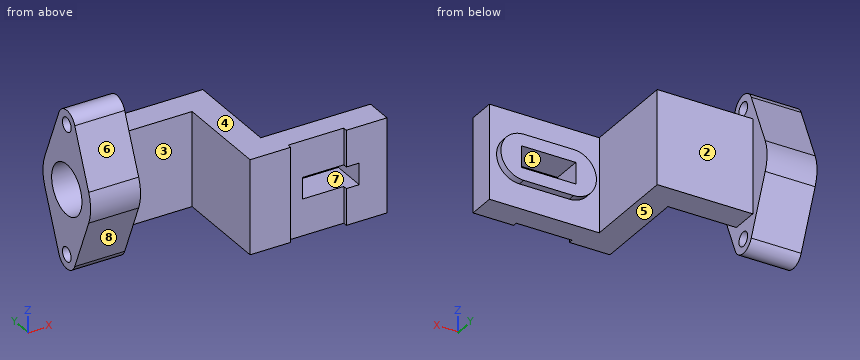
```python
from build123d import *

# Parameters (mm, degrees)
BOSS_EXTRUDE1_DEPTH = 33
BOSS_EXTRUDE2_DEPTH = 5
SKETCH3_W           = 38
SKETCH3_H           = 15
CUT_EXTRUDE1_DEPTH  = 119.949569146
SKETCH4_R           = 5
BOSS_EXTRUDE3_DEPTH = 35
HOLE1_D             = 35
HOLE1_DEPTH         = 34


with BuildPart() as part:
    # Sketch1 → Boss-Extrude1 (new, symmetric)
    with BuildSketch(Plane.XY):
        Polygon((-96, 86), (-29, 86), (-29, 19), (48, 19), (48, 0), (19.5, 0), (19.5, 3), (-19.5, 3), (-19.5, 0), (-48, 0), (-48, 67), (-96, 67), align=None)
    extrude(amount=BOSS_EXTRUDE1_DEPTH, both=True)

    # Sketch2 → Boss-Extrude2 (add)
    with BuildSketch(Plane(origin=(0, 19, 0), x_dir=(1, 0, 0), z_dir=(0, 1, 0))):
        with BuildLine():
            Line((-8, 16), (27, 16))
            ThreePointArc((27, 16), (43, 0), (27, -16))
            Line((27, -16), (-8, -16))
            ThreePointArc((-8, -16), (-24, 0), (-8, 16))
        make_face()
    extrude(amount=BOSS_EXTRUDE2_DEPTH)

    # Sketch3 → Cut-Extrude1 (cut, through all)
    with BuildSketch(Plane(origin=(0, 24, 0), x_dir=(1, 0, 0), z_dir=(0, 1, 0))):
        with Locations((9.5, 0)):
            Rectangle(SKETCH3_W, SKETCH3_H)
    extrude(amount=-CUT_EXTRUDE1_DEPTH, mode=Mode.SUBTRACT)

    # Sketch4 → Boss-Extrude3 (add)
    with BuildSketch(Plane.ZY.offset(96)):
        with BuildLine():
            Line((-48.888888889, 84.21284664), (-10.694444444, 100.33532826))
            ThreePointArc((-10.694444444, 100.33532826), (0, 102.5), (10.694444444, 100.33532826))
            Line((10.694444444, 100.33532826), (48.888888889, 84.21284664))
            ThreePointArc((48.888888889, 84.21284664), (55, 75), (48.888888889, 65.78715336))
            Line((48.888888889, 65.78715336), (10.694444444, 49.66467174))
            ThreePointArc((10.694444444, 49.66467174), (0, 47.5), (-10.694444444, 49.66467174))
            Line((-10.694444444, 49.66467174), (-48.888888889, 65.78715336))
            ThreePointArc((-48.888888889, 65.78715336), (-55, 75), (-48.888888889, 84.21284664))
        make_face()
        with Locations((-45, 75)):
            Circle(SKETCH4_R, mode=Mode.SUBTRACT)
        with Locations((45, 75)):
            Circle(SKETCH4_R, mode=Mode.SUBTRACT)
    extrude(amount=BOSS_EXTRUDE3_DEPTH)

    # Hole1
    with Locations(Plane.ZY.offset(131)):
        with Locations((0, 75)):
            Hole(HOLE1_D / 2, depth=HOLE1_DEPTH)


solid = part.part
```
Can you work these out from the model? Positions are in its coordinate system, mm. Face numbers are marked on the shaded views. A direction names the side the tool comes from. Coordinates: 2 decimals unless noted, no trailing zeros. Loops run counter-clockwise (first coordinate to the right, second up) from the corner with the lowest first, then second, coordinate; pieces in that order, holes last.
1) Imagine slicing it at A-A on z = 0. List the corners of the cut face in (x, y) for me, plus the area to 3 significant figures.
2) Which directions (+Z, -Z, +X, -X, +Y, -Y) give clear straight access to the entire face, cutting with the end or side of a thin tool? Please do the marked faces 1, 2, 3, 4 and 5.
3) Thinking about a two-plate mould opening in Z: for the marked faces 6, 7 and 8, which applies, pulls with the +Z half, pulls with the -Z half, needs draft (parallel to the pull), parting line crosses it, or undercut?
4) Imagine slicing it at B-B on x = 2.5. List the corners of the cut face in (y, z) for me, plus the area to 3 significant figures.
5) Imagine slicing it at C-C on y = 75. List the corners of the cut face in (x, z) for me, plus the area to 3 significant figures.
6) I need wall thicknesses on probe 1 along Y at (x, z) = (-123, 0); probe 2 along X at (y, z) = (31, 29.5); probe 3 along Y at (x, z) = (-63.5, -8). Which ranges of each line are inside material? Lowest first, please.
7) Imagine slicing it at D-D on x = -113.5. List the corners of the cut face in (y, z) for me, plus the area to 3 significant figures.
8) For pin 1 (12 mm diameter, centred on x = 3.5, y = 26, fed in from -Z); pin 2 (8 mm diameter, centred on y = 46.5, z = 31.5, fed in from +X); pin 3 (14.5 mm diameter, centred on x = -72.5, z = 11, fed in from -Y); pin 4 (8 mm diameter, centred on x = 10.5, z = -39.5, fed in from -Y), each with a flat end and sliding along its axis, tell me the tip position at first contact or that it passes through.
Completed:
1. outline: (-131, 47.5) - (-96, 47.5) - (-96, 67) - (-48, 67) - (-48, 0) - (-19.5, 0) - (-19.5, 3) - (-9.5, 3) - (-9.5, 24) - (-24, 24) - (-24, 19) - (-29, 19) - (-29, 86) - (-96, 86) - (-96, 102.5) - (-131, 102.5) - (-131, 92.5) - (-97, 92.5) - (-97, 57.5) - (-131, 57.5) - close; (28.5, 0) - (48, 0) - (48, 19) - (43, 19) - (43, 24) - (28.5, 24) - close
1. area: 4,140 mm2
2. face 1: +Y, -Y
2. face 2: +Z, -Z, +X, +Y
2. face 3: +Z, -Z, -Y
2. face 4: +Z, +X, +Y, -Y
2. face 5: -Z, +X, +Y, -Y
3. face 6: pulls with the +Z half
3. face 7: undercut
3. face 8: pulls with the -Z half
4. outline: (3, -33) - (19, -33) - (19, -16) - (24, -16) - (24, -7.5) - (3, -7.5) - close; (3, 7.5) - (24, 7.5) - (24, 16) - (19, 16) - (19, 33) - (3, 33) - close
4. area: 901 mm2
5. outline: (-131, -55) - (-96, -55) - (-96, -50) - (-131, -50) - close; (-131, -40) - (-96, -40) - (-96, -33) - (-29, -33) - (-29, 33) - (-96, 33) - (-96, 40) - (-131, 40) - (-131, 17.5) - (-97, 17.5) - (-97, -17.5) - (-131, -17.5) - close; (-131, 50) - (-96, 50) - (-96, 55) - (-131, 55) - close
5. area: 6,380 mm2
6. probe 1: y = 47.5 to 57.5, 92.5 to 102.5
6. probe 2: x = -48 to -29
6. probe 3: y = 67 to 86
7. outline: (49.66, -10.69) - (65.79, -48.89) arc R10 ccw to (84.21, -48.89) - (100.34, -10.69) arc R27.5 ccw to (100.34, 10.69) - (84.21, 48.89) arc R10 ccw to (65.79, 48.89) - (49.66, 10.69) arc R27.5 ccw to start; hole circle Ø35 at (75, 0); hole circle Ø10 at (75, -45); hole circle Ø10 at (75, 45)
7. area: 2,830 mm2
8. pin 1: stops at z = -16
8. pin 2: stops at x = -29
8. pin 3: stops at y = 67
8. pin 4: passes through
